Check sheet for the modelled part. Datum: model origin and axes. Units: mm. Round coordinates to 2 decimals unless told otherwise and drop trailing zeros. Order: outer loops, then holes, each group sorted by start corner. A loop starts at its lowest first (then second) coordinate and runs counter-clockwise, first axis right, second up.
(1) Sectioned sample at C-C, the plane y = -123. Enter the section's corners in (x, z), and give its area (4 significant figures).
(2) Sectioned sample at B-B, the plane y = 148.5. Enter the section's corners in (x, z), and give its area (3 significant figures).
(3) Thickness scan on probe 1 along X at (y, z) = (-137.5, 1.2); probe 2 along X at (y, z) = (-69, 1.25); probe 3 along Y at (x, z) = (-29, 0.5). Record the ranges inside material, lowest first.
(4) Sectioned sample at D-D, the plane x = 0. Enter the section's corners in (y, z), and give its area (3 significant figures).
(5) Sectioned sample at A-A, the plane x = -39. Enter the section's corners in (y, z), and give its area (3 significant figures).
Autodesk Inventor part; units mm, degrees
ref_plane "YZ Plane" through (0, 0, 0) normal (1, 0, 0) x (0, 1, 0)
ref_plane "XZ Plane" through (0, 0, 0) normal (0, 1, 0) x (-1, 0, 0)
ref_plane "XY Plane" through (0, 0, 0) normal (0, 0, 1) x (1, 0, 0)
sketch "Skizze1" plane through (0, 0, 0) normal (0, 0, 1) x (1, 0, 0)
  line L0 (-135.1, 0) -> (135.1, 0)
  line L1 (0, -215.3) -> (0, 220.8)
  line L2 (15, 140.5) -> (15, 158.5)
  line L3 (15, 158.5) -> (-15, 158.5)
  line L4 (-15, 158.5) -> (-15, 140.5)
  line L5 (-15, 140.5) -> (-96.5, 140.5)
  line L6 (-96.5, 140.5) -> (-96.5, -153)
  line L7 (-96.5, -153) -> (96.5, -153)
  line L8 (96.5, -153) -> (96.5, 140.5)
  line L9 (96.5, 140.5) -> (15, 140.5)
  circle A0 centre (86.5, 78) radius 2.5
  circle A1 centre (-86.5, 78) radius 2.5
  circle A2 centre (-86.5, -89) radius 2.5
  circle A3 centre (86.5, -89) radius 2.5
  arc A4 (-71.5, 132) -> (-76.5, 132) centre (-74, 132) ccw
  line L10 (-76.5, 132) -> (-76.5, 101.5)
  arc A5 (-76.5, 101.5) -> (-71.5, 101.5) centre (-74, 101.5) ccw
  line L11 (-71.5, 101.5) -> (-71.5, 132)
  arc A6 (76.5, 132) -> (71.5, 132) centre (74, 132) ccw
  line L12 (76.5, 132) -> (76.5, 101.5)
  arc A7 (71.5, 101.5) -> (76.5, 101.5) centre (74, 101.5) ccw
  line L13 (71.5, 101.5) -> (71.5, 132)
  line L14 (-80.5, 75) -> (80.5, 75)
  line L15 (80.5, 75) -> (80.5, 0)
  line L16 (80.5, 0) -> (-80.5, 0)
  line L17 (-80.5, 0) -> (-80.5, 75)
  circle A8 centre (29, -20) radius 1.25
  circle A9 centre (-29, -20) radius 1.25
  circle A10 centre (-29, -69) radius 1.25
  circle A11 centre (29, -69) radius 1.25
  arc A12 (-71.5, -112.5) -> (-76.5, -112.5) centre (-74, -112.5) ccw
  line L18 (-76.5, -112.5) -> (-76.5, -143)
  arc A13 (-76.5, -143) -> (-71.5, -143) centre (-74, -143) ccw
  line L19 (-71.5, -143) -> (-71.5, -112.5)
  arc A14 (76.5, -112.5) -> (71.5, -112.5) centre (74, -112.5) ccw
  line L20 (76.5, -112.5) -> (76.5, -143)
  arc A15 (71.5, -143) -> (76.5, -143) centre (74, -143) ccw
  line L21 (71.5, -143) -> (71.5, -112.5)
  circle A16 centre (0, 148.5) radius 5
  point P0 (0, 0)
  dimension "d0" = 30
  dimension "d1" = 193
  dimension "d2" = 293.5
  dimension "d3" = 65.5
  dimension "d4" = 75
  dimension "d5" = 16
  dimension "d6" = 16
  dimension "d7" = 65.5
  dimension "d9" = 148
  dimension "d10" = 5
  dimension "d11" = 2.5
  dimension "d12" = 2.5
  dimension "d13" = 30.5
  dimension "d14" = 8.5
  dimension "d15" = 5
  dimension "d16" = 30.5
  dimension "d17" = 2.5
  dimension "d18" = 2.5
  dimension "d19" = 143
  dimension "d20" = 6
  dimension "d21" = 3
  dimension "d22" = 6
  dimension "d23" = 3
  dimension "d24" = 75
  dimension "d25" = 167
  dimension "d26" = 10
  dimension "d27" = 167
  dimension "d28" = 10
  dimension "d29" = 20
  dimension "d30" = 8.5
  dimension "d31" = 81.5
  dimension "d32" = 58
  dimension "d33" = 49
  dimension "d34" = 58
  dimension "d35" = 49
  dimension "d36" = 67.5
  dimension "d37" = 67.5
  dimension "d38" = 67.5
  dimension "d39" = 20
  dimension "d40" = 84
  dimension "d41" = 5
  dimension "d42" = 5
  dimension "d43" = 2.5
  dimension "d44" = 2.5
  dimension "d45" = 2.5
  dimension "d46" = 2.5
  dimension "d47" = 5
  dimension "d48" = 5
  dimension "d49" = 2.5
  dimension "d50" = 2.5
  dimension "d51" = 2.5
  dimension "d52" = 2.5
  dimension "d53" = 30.5
  dimension "d54" = 30.5
  dimension "d55" = 5
  dimension "d56" = 5
  dimension "d57" = 10
  dimension "d58" = 10
  dimension "d59" = 22.5
  dimension "d60" = 22.5
  dimension "d61" = 22.5
  dimension "d62" = 22.5
  dimension "d63" = 143
  dimension "d65" = 18
extrude "Extrusion1" add sketch "Skizze1" along normal blind 1.5 contours L6 L5 L4 L3 L1 A16 L14 L17 L0 | L0 L1 L7 L6 | L0 L8 L7 L1 | L15 L14 L1 A16 L3 L2 L9 L8 L0
properties part number "Innengehäuse"
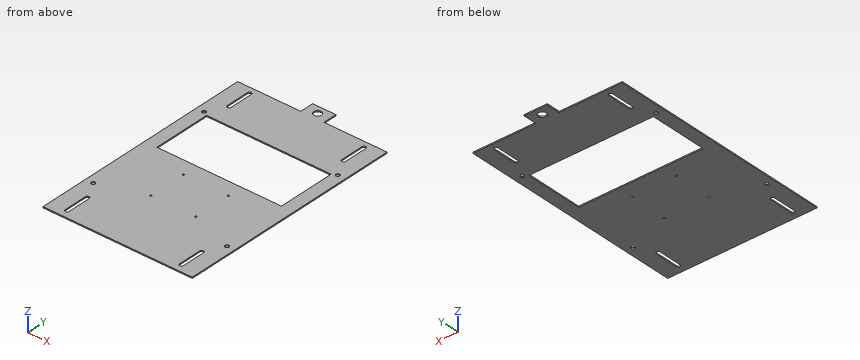
Derived:
1. outline: (-96.5, 0) - (-76.5, 0) - (-76.5, 1.5) - (-96.5, 1.5) - close; (-71.5, 0) - (71.5, 0) - (71.5, 1.5) - (-71.5, 1.5) - close; (76.5, 0) - (96.5, 0) - (96.5, 1.5) - (76.5, 1.5) - close
1. area: 274.5 mm2
2. outline: (-15, 0) - (-5, 0) - (-5, 1.5) - (-15, 1.5) - close; (5, 0) - (15, 0) - (15, 1.5) - (5, 1.5) - close
2. area: 30.0 mm2
3. probe 1: x = -96.5 to -76.5, -71.5 to 71.5, 76.5 to 96.5
3. probe 2: x = -96.5 to -30.25, -27.75 to 27.75, 30.25 to 96.5
3. probe 3: y = -153 to -70.25, -67.75 to -21.25, -18.75 to 0, 75 to 140.5
4. outline: (-153, 0) - (0, 0) - (0, 1.5) - (-153, 1.5) - close; (75, 0) - (143.5, 0) - (143.5, 1.5) - (75, 1.5) - close; (153.5, 0) - (158.5, 0) - (158.5, 1.5) - (153.5, 1.5) - close
4. area: 340 mm2
5. outline: (-153, 0) - (0, 0) - (0, 1.5) - (-153, 1.5) - close; (75, 0) - (140.5, 0) - (140.5, 1.5) - (75, 1.5) - close
5. area: 328 mm2
